from build123d import *

# Parameters (mm, degrees)
F0_W          = 116
F0_H          = 55
F1_DEPTH      = 15.2
F2_R          = 7
F3_W          = 10
F3_H          = 15.2
F4_DEPTH      = 5
F4_DEPTH_BACK = 10


with BuildPart() as f1:
    # F0 (on Top) → F1 (new body)
    with BuildSketch(Plane.XY):
        Rectangle(F0_W, F0_H)
    extrude(amount=F1_DEPTH)

    # F2
    f2_edges = [f1.edges().sort_by_distance(p)[0] for p in [
        (58, 0, 15.2),
        (58, 0, 0),
        (-58, 0, 15.2),
        (-58, 0, 0),
    ]]
    fillet(f2_edges, radius=F2_R)

    # F3 (on face) → F4 (join, two sides)
    with BuildSketch(Plane.YZ.offset(58)) as f4_sk:
        with Locations((-22.5, 7.6)):
            Rectangle(F3_W, F3_H)
    extrude(amount=F4_DEPTH)
    extrude(f4_sk.sketch, amount=-F4_DEPTH_BACK)


solid = f1.part
Check sheet for the modelled part. Datum: model origin and axes. Units: mm. A direction names the side the tool comes from. Give positions to 0.01 mm unless a question says otherwise; leave off trailing zeros. Write each loop counter-clockwise with the first axis right and the second up, starting at its lowest first coordinate (ties: lowest second). Pieces come first, ordered by that corner, then holes. Notation, with made-up numbers: M 8.25,52.5 L 28.25,52.5 A28 ccw 28.25,74.5 Z; hole C 13.5,72 d11. An arc over 180 degrees is marked long. Use one line per item in the form item = value.
(1) Section check B-B on x = 54. Record the boundary of the cut face in (y, z), plus the area to 3 significant figures.
Answer block:
outline = M -27.5,0 L -17.5,0 L -17.5,0.68 L 27.5,0.68 L 27.5,14.52 L -17.5,14.52 L -17.5,15.2 L -27.5,15.2 Z
area = 775 mm2
(2) Section check A-A on y = 8.5. Record the boundary of the cut face in (x, z), plus the area to 3 significant figures.
Answer block:
outline = M -58,7 A7 ccw -51,0 L 51,0 A7 ccw 58,7 L 58,8.2 A7 ccw 51,15.2 L -51,15.2 A7 ccw -58,8.2 Z
area = 1,720 mm2
(3) Depth check by flat-ended pin: P1, Ø8, axis at y = 5.5, z = 4.5, coming from the +X side. Enter the tip coordinate at first touch or a pass-through.
Answer block:
P1 = 58
(4) Section check C-C on z = 4. Record the boundary of the cut face in (x, y).
Answer block:
outline = M -57.32,-27.5 L 63,-27.5 L 63,-17.5 L 57.32,-17.5 L 57.32,27.5 L -57.32,27.5 Z
(5) Material ranges on line 1 along X through (y, z) = (0, 7.75); line 2 along X through (y, z) = (18.5, 5.5), recorded low to high.
Answer block:
line_1 = -58 to 58
line_2 = -57.84 to 57.84
(6) Tool access check on faces 1 (the flat face through (63, -23, 8)), 2 (the cylindrical face through (56, 5.3, 13.1)), 3 (the cylindrical face through (56, 5.3, 2.1)). Record the directions out of +Z, -Z, +X, -X, +Y, -Y that give a thin tool (end or side, any length) a straight path to the whole face; none if there is none.
Answer block:
face_1 = +Z, -Z, +X, +Y, -Y
face_2 = +Z, +X, +Y
face_3 = -Z, +X, +Y
